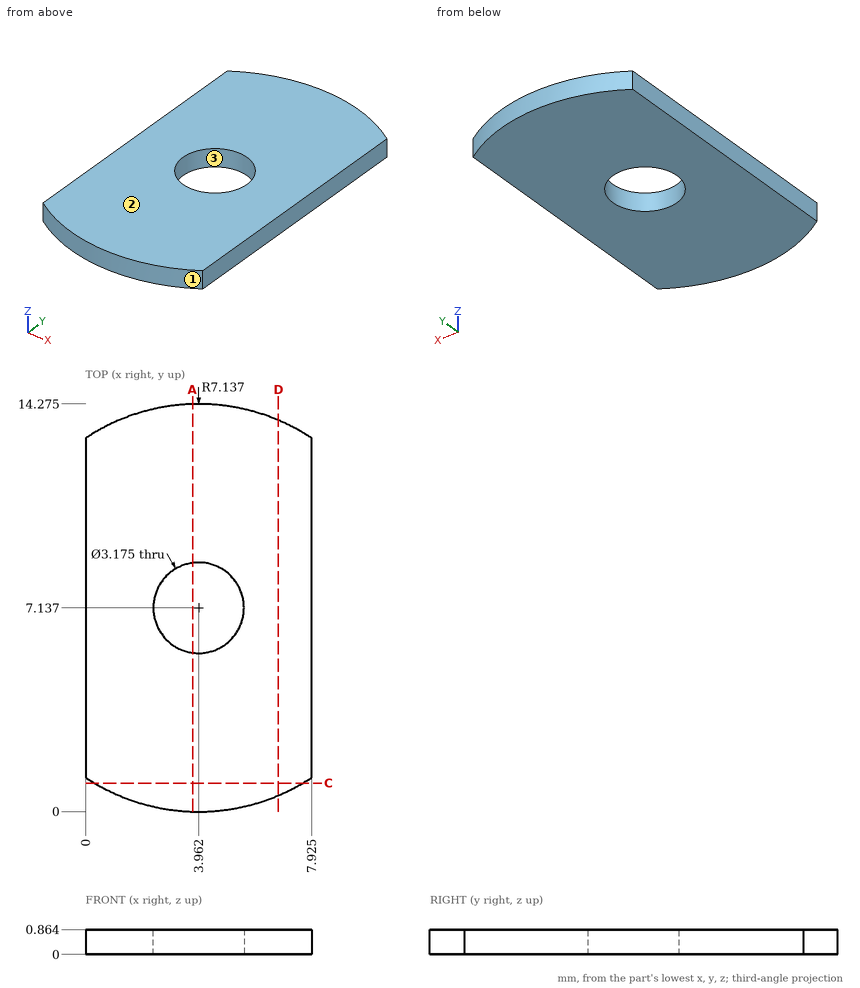
Design review of the part shown in the three views and the two pictorial views. Dimensions are in mm from the part's minimum x, y and z. Give positions to 0.01 mm unless a question says otherwise; leave off trailing zeros. Write each loop counter-clockwise with the first axis right and the second up, starting at its lowest first coordinate (ties: lowest second). Pieces come first, ordered by that corner, then holes. Notation, with made-up numbers: (15.5, 61) - (70.5, 61) arc R13 ccw to (70.5, 68) - close; hole circle Ø5 at (61.25, 88.5). An arc over 180 degrees is marked (long way). Return JSON: item names as keys, results as strings. Group by question number.
(1) We need section C-C, the plane y = 1. Give the boundary of the cut face in (x, z).
(2) We need section A-A, the plane x = 3.75. Give the boundary of the cut face in (y, z).
(3) To check wall thickness, follow probe 1 along Y at (x, z) = (3.25, 0.3) (1 decimal); probe 2 along Y at (x, z) = (4.5, 0.25) (1 decimal); probe 3 along X at (y, z) = (7, 0.3) (1 decimal). State the ranges of each line that lie inside material, in increasing order.
(4) We need section D-D, the plane x = 6.75. Give the boundary of the cut face in (y, z).
(5) Mouldability with a two-part tool opening along X and no side actions: class the marked faces 1, 2 and 3 as +X half, -X half, draft (parallel to the pull), parting line (faces both ways), or undercut.
Reported:
{
 "1": {"outline": "(0.32, 0) - (7.61, 0) - (7.61, 0.86) - (0.32, 0.86) - close"},
 "2": {"outline": "(0, 0) - (5.56, 0) - (5.56, 0.86) - (0, 0.86) - close; (8.71, 0) - (14.27, 0) - (14.27, 0.86) - (8.71, 0.86) - close"},
 "3": {"probe 1": "y = 0 to 5.7, 8.6 to 14.2", "probe 2": "y = 0 to 5.6, 8.6 to 14.3", "probe 3": "x = 0 to 2.4, 5.5 to 7.9"},
 "4": {"outline": "(0.57, 0) - (13.71, 0) - (13.71, 0.86) - (0.57, 0.86) - close"},
 "5": {"face 1": "parting line", "face 2": "draft", "face 3": "undercut"}
}
